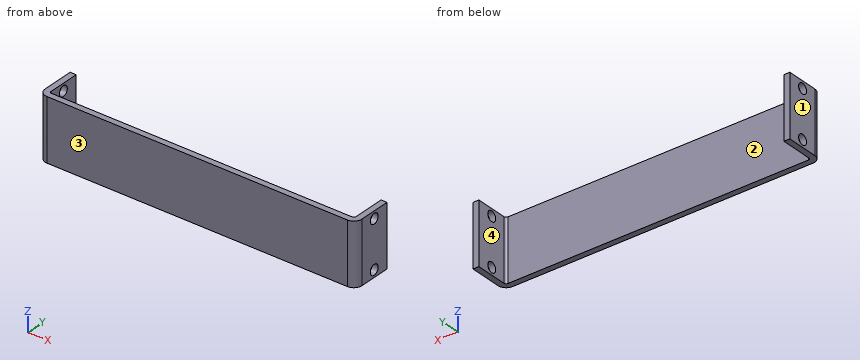
from build123d import *

# Parameters (mm, degrees)
SKETCH_2_W             = 128.39072245
SKETCH_2_H             = 20.758785388
SKETCH_2_R             = 1.7
SM_BASE_FLANGE_1_DEPTH = 2
OTHER_START            = -15.144216699
OTHER_1_DEPTH          = 20.758785388
OTHER_START_2          = -11.014823905
OTHER_1_2_DEPTH        = 12.4999998
OTHER_1_3_DEPTH        = 0.729392594
OTHER_START_3          = 4.885176095
OTHER_1_4_DEPTH        = 0.729392594
OTHER_START_4          = -14.414824105
OTHER_1_5_DEPTH        = 19.3000002
OTHER_START_5          = -109.217240912
OTHER_1_6_OUTLINE_R    = 1.7
OTHER_1_6_DEPTH        = 106.86392245


with BuildPart() as part:
    # 基体-法兰1: sheet metal written as solids
    # Sketch 2 → 基体-法兰1 (new body)
    with BuildSketch(Plane(origin=(0, 0, 0), x_dir=(1, 0, 0), z_dir=(0, 1, 0))):
        with Locations((-55.785279687, 4.764824005)):
            Rectangle(SKETCH_2_W, SKETCH_2_H)
        with Locations(Location((2.910081538, 12.714824005, 0), (0, 0, 270))):
            Circle(SKETCH_2_R, mode=Mode.SUBTRACT)
        with Locations(Location((2.910081538, -3.185175995, 0), (0, 0, 270))):
            Circle(SKETCH_2_R, mode=Mode.SUBTRACT)
        with Locations(Location((-114.480640912, -3.185175995, 0), (0, 0, 90))):
            Circle(SKETCH_2_R, mode=Mode.SUBTRACT)
        with Locations(Location((-114.480640912, 12.714824005, 0), (0, 0, 90))):
            Circle(SKETCH_2_R, mode=Mode.SUBTRACT)
    extrude(amount=-SM_BASE_FLANGE_1_DEPTH)

    # Other 1: read off the stored shape, not the designer's step
    # Other 1 outline → Other 1 (cut)
    with BuildSketch(Plane.XY.offset(OTHER_START)):
        with BuildLine():
            Line((-119.980640912, -2), (-106.480640912, -2))
            ThreePointArc((-106.480640912, -2), (-108.134908121, -1.443395312), (-109.11624331, 0))
            Line((-109.11624331, 0), (-119.980640912, 0))
            Line((-119.980640912, 0), (-119.980640912, -2))
        make_face()
        with BuildLine():
            ThreePointArc((-2.454316064, 0), (-3.435651253, -1.443395312), (-5.089918462, -2))
            Line((-5.089918462, -2), (8.410081538, -2))
            Line((8.410081538, -2), (8.410081538, 0))
            Line((8.410081538, 0), (-2.454316064, 0))
        make_face()
    extrude(amount=OTHER_1_DEPTH, mode=Mode.SUBTRACT)

    # Other 1 2 outline → Other 1 2 (add)
    with BuildSketch(Plane.XY.offset(OTHER_START_2)):
        with BuildLine():
            ThreePointArc((-109.217240912, 0.7366), (-109.191873941, 0.364854094), (-109.11624331, 0))
            Line((-109.11624331, 0), (-106.480640912, 0))
            ThreePointArc((-106.480640912, 0), (-107.001495767, 0.215745145), (-107.217240912, 0.7366))
            Line((-107.217240912, 0.7366), (-107.217240912, 11.508755099))
            Line((-107.217240912, 11.508755099), (-109.217240912, 11.508755099))
            Line((-109.217240912, 11.508755099), (-109.217240912, 0.7366))
        make_face()
        with BuildLine():
            Line((-5.089918462, 0), (-2.454316064, 0))
            ThreePointArc((-2.454316064, 0), (-2.378685433, 0.364854094), (-2.353318462, 0.7366))
            Line((-2.353318462, 0.7366), (-2.353318462, 11.508755099))
            Line((-2.353318462, 11.508755099), (-4.353318462, 11.508755099))
            Line((-4.353318462, 11.508755099), (-4.353318462, 0.7366))
            ThreePointArc((-4.353318462, 0.7366), (-4.569063607, 0.215745145), (-5.089918462, 0))
        make_face()
    extrude(amount=OTHER_1_2_DEPTH)

    # Other 1 3 outline → Other 1 3 (add)
    with BuildSketch(Plane.XY.offset(OTHER_START)):
        with BuildLine():
            ThreePointArc((-109.217240912, 0.7366), (-109.191873941, 0.364854094), (-109.11624331, 0))
            Line((-109.11624331, 0), (-106.480640912, 0))
            ThreePointArc((-106.480640912, 0), (-107.001495767, 0.215745145), (-107.217240912, 0.7366))
            Line((-107.217240912, 0.7366), (-107.217240912, 11.508755099))
            Line((-107.217240912, 11.508755099), (-109.217240912, 11.508755099))
            Line((-109.217240912, 11.508755099), (-109.217240912, 0.7366))
        make_face()
        with BuildLine():
            Line((-5.089918462, 0), (-2.454316064, 0))
            ThreePointArc((-2.454316064, 0), (-2.378685433, 0.364854094), (-2.353318462, 0.7366))
            Line((-2.353318462, 0.7366), (-2.353318462, 11.508755099))
            Line((-2.353318462, 11.508755099), (-4.353318462, 11.508755099))
            Line((-4.353318462, 11.508755099), (-4.353318462, 0.7366))
            ThreePointArc((-4.353318462, 0.7366), (-4.569063607, 0.215745145), (-5.089918462, 0))
        make_face()
    extrude(amount=OTHER_1_3_DEPTH)

    # Other 1 4 outline → Other 1 4 (add)
    with BuildSketch(Plane.XY.offset(OTHER_START_3)):
        with BuildLine():
            ThreePointArc((-109.217240912, 0.7366), (-109.191873941, 0.364854094), (-109.11624331, 0))
            Line((-109.11624331, 0), (-106.480640912, 0))
            ThreePointArc((-106.480640912, 0), (-107.001495767, 0.215745145), (-107.217240912, 0.7366))
            Line((-107.217240912, 0.7366), (-107.217240912, 11.508755099))
            Line((-107.217240912, 11.508755099), (-109.217240912, 11.508755099))
            Line((-109.217240912, 11.508755099), (-109.217240912, 0.7366))
        make_face()
        with BuildLine():
            Line((-5.089918462, 0), (-2.454316064, 0))
            ThreePointArc((-2.454316064, 0), (-2.378685433, 0.364854094), (-2.353318462, 0.7366))
            Line((-2.353318462, 0.7366), (-2.353318462, 11.508755099))
            Line((-2.353318462, 11.508755099), (-4.353318462, 11.508755099))
            Line((-4.353318462, 11.508755099), (-4.353318462, 0.7366))
            ThreePointArc((-4.353318462, 0.7366), (-4.569063607, 0.215745145), (-5.089918462, 0))
        make_face()
    extrude(amount=OTHER_1_4_DEPTH)

    # Other 1 5 outline → Other 1 5 (add)
    with BuildSketch(Plane.XY.offset(OTHER_START_4)):
        with BuildLine():
            ThreePointArc((-4.353318462, 0.7366), (-4.569063607, 0.215745145), (-5.089918462, 0))
            Line((-5.089918462, 0), (-2.454316064, 0))
            ThreePointArc((-2.454316064, 0), (-2.378685433, 0.364854094), (-2.353318462, 0.7366))
            Line((-2.353318462, 0.7366), (-2.353318462, 11.508755099))
            Line((-2.353318462, 11.508755099), (-4.353318462, 11.508755099))
            Line((-4.353318462, 11.508755099), (-4.353318462, 0.7366))
        make_face()
        with BuildLine():
            ThreePointArc((-109.217240912, 0.7366), (-109.191873941, 0.364854094), (-109.11624331, 0))
            Line((-109.11624331, 0), (-106.480640912, 0))
            ThreePointArc((-106.480640912, 0), (-107.001495767, 0.215745145), (-107.217240912, 0.7366))
            Line((-107.217240912, 0.7366), (-107.217240912, 11.508755099))
            Line((-107.217240912, 11.508755099), (-109.217240912, 11.508755099))
            Line((-109.217240912, 11.508755099), (-109.217240912, 0.7366))
        make_face()
    extrude(amount=OTHER_1_5_DEPTH)

    # Other 1 6 outline → Other 1 6 (cut)
    with BuildSketch(Plane.YZ.offset(OTHER_START_5)):
        with Locations((6.008755099, -12.714824005)):
            Circle(OTHER_1_6_OUTLINE_R)
        with Locations((6.008755099, 3.185175995)):
            Circle(OTHER_1_6_OUTLINE_R)
    extrude(amount=OTHER_1_6_DEPTH, mode=Mode.SUBTRACT)


solid = part.part
The listing builds one solid part. Answer for the finished solid, in the listing's coordinates (mm). Face numbers are marked on the shaded views. Round coordinates to 2 decimals unless told otherwise and drop trailing zeros. Write each loop counter-clockwise with the first axis right and the second up, starting at its lowest first coordinate (ties: lowest second). Pieces come first, ordered by that corner, then holes. Notation, with made-up numbers: (33.5, 44.5) - (84.5, 44.5) arc R25 cw to (84.5, 78.5) - close; hole circle Ø11 at (52.5, -21.75). An arc over 180 degrees is marked (long way). Use one line per item in the form item = value. Start each with the question number.
Item 1: A flat-ended cylindrical pin translates along its axis: pin 1 Ø10.5 at (x, z) = (-42.5, -1.5) entering from +Y. Find the tip coordinate at first contact, or state that the pin passes through.
Item 2: Determine the mould class of the marked faces 1, 2, 3 and 4 for opening direction X: +X half, -X half, draft (parallel to the pull), parting line (faces both ways), or undercut.
Item 3: A cutting plane is placed at A-A (y = 2.75). Write down the section's boundary in (x, z), plus the area to 3 significant figures.
Item 4: Find the intervals of material crossed by line 1 (X direction, y = 5.25, z = -9); line 2 (Y direction, x = -39.5, z = -12); line 3 (X direction, y = -0.25, z = -10), in increasing order. Write a range as [from, to].
Item 5: A cutting plane is placed at C-C (x = -50). Write down the section's boundary in (y, z).
Item 6: A cutting plane is placed at B-B (z = -0.25). Write down the section's boundary in (x, y).
The answers:
q1.pin_1 = 0
q2.face_1 = -X half
q2.face_2 = undercut
q2.face_3 = draft
q2.face_4 = undercut
q3.outline = (-109.22, -15.14) - (-107.22, -15.14) - (-107.22, 5.61) - (-109.22, 5.61) - close; (-4.35, -15.14) - (-2.35, -15.14) - (-2.35, 5.61) - (-4.35, 5.61) - close
q3.area = 83.0 mm^2
q4.line_1 = [-109.22, -107.22], [-4.35, -2.35]
q4.line_2 = [-2, 0]
q4.line_3 = [-109.03, -2.54]
q5.outline = (-2, -15.14) - (0, -15.14) - (0, 5.61) - (-2, 5.61) - close
q6.outline = (-109.22, 0.74) arc R2.74 ccw to (-106.48, -2) - (-5.09, -2) arc R2.74 ccw to (-2.35, 0.74) - (-2.35, 11.51) - (-4.35, 11.51) - (-4.35, 0.74) arc R0.74 cw to (-5.09, 0) - (-106.48, 0) arc R0.74 cw to (-107.22, 0.74) - (-107.22, 11.51) - (-109.22, 11.51) - close
